Source: CAD feature listing. Evaluate the final solid. Frame: model axes, mm. Face numbers are marked on the shaded views. A direction names the side the tool comes from. Round coordinates to 2 decimals unless told otherwise and drop trailing zeros. Order: outer loops, then holes, each group sorted by start corner. A loop starts at its lowest first (then second) coordinate and runs counter-clockwise, first axis right, second up. Notation, with made-up numbers: M 41,-1 L 87,-1 A10 cw 87,13 Z; hole C 83.5,87 d6. An arc over 180 degrees is marked long. Answer in a Markdown table with one row per item. Add a question column.
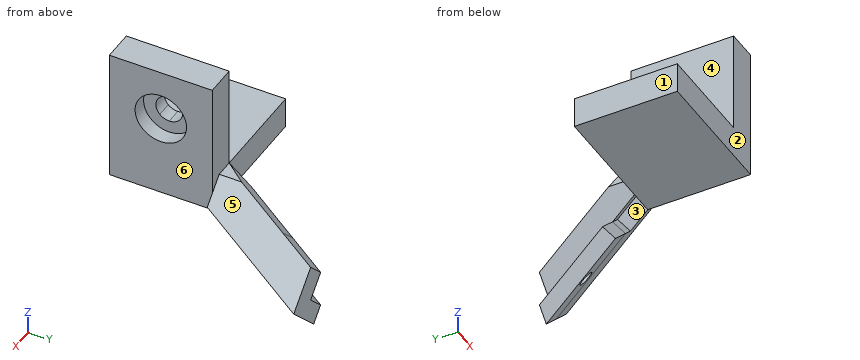
```python
from build123d import *

# Parameters (mm, degrees)
EXTRUDE_2_DEPTH     = 20
CUT_EXTRUDE_1_DEPTH = 20
SKETCH_3_R          = 5
CUT_EXTRUDE_2_DEPTH = 3
SKETCH_4_W          = 6
SKETCH_4_H          = 6
EXTRUDE_3_DEPTH     = 84
CUT_EXTRUDE_3_DEPTH = 84
CUT_EXTRUDE_4_DEPTH = 84
CUT_EXTRUDE_5_DEPTH = 84
SKETCH_9_R          = 1.5
EXTRUDE_4_DEPTH     = 3
CUT_EXTRUDE_6_DEPTH = 6
CUT_EXTRUDE_7_DEPTH = 2.5


with BuildPart() as part:
    # 草图1 → 凸台-拉伸2 (new body)
    with BuildSketch(Plane(origin=(0, 0, 0), x_dir=(1, 0, 0), z_dir=(0, 1, 0))):
        Polygon((0, 0), (0, -20), (6, -20), (6, 6), (-20, 6), (-20, 0), align=None)
    extrude(amount=EXTRUDE_2_DEPTH)

    # 草图2 → 切除-拉伸1 (cut)
    with BuildSketch(Plane(origin=(6, 0, 0), x_dir=(0, 0, -1), z_dir=(1, 0, 0))):
        with BuildLine():
            ThreePointArc((-11.838477631, 11.838477631), (-11.838477631, 8.161522369), (-8.161522369, 8.161522369))
            Line((-8.161522369, 8.161522369), (-11.838477631, 11.838477631))
        make_face()
        with BuildLine():
            Line((-11.838477631, 11.838477631), (-8.161522369, 8.161522369))
            ThreePointArc((-8.161522369, 8.161522369), (-7.597913215, 9.005023076), (-7.4, 10))
            ThreePointArc((-7.4, 10), (-9.005023076, 12.402086785), (-11.838477631, 11.838477631))
        make_face()
    extrude(amount=-CUT_EXTRUDE_1_DEPTH, mode=Mode.SUBTRACT)

    # 草图3 → 切除-拉伸2 (cut)
    with BuildSketch(Plane(origin=(6, 0, 0), x_dir=(0, 0, -1), z_dir=(1, 0, 0))):
        with Locations((-10, 10)):
            Circle(SKETCH_3_R)
    extrude(amount=-CUT_EXTRUDE_2_DEPTH, mode=Mode.SUBTRACT)

    # 草图4 → 凸台-拉伸3 (add)
    with BuildSketch(Plane(origin=(0, 20, 0), x_dir=(1, 0, 0), z_dir=(0, 1, 0))):
        Polygon((65.39696962, 65.39696962), (6, 6), (7.767766953, 4.232233047), (67.164736573, 63.629202667), align=None)
        Polygon((4.232233047, 7.767766953), (6, 6), (65.39696962, 65.39696962), (63.629202667, 67.164736573), align=None)
        Polygon((0, 6), (6, 6), (4.232233047, 7.767766953), (0, 12), align=None)
        with Locations((3, 3)):
            Rectangle(SKETCH_4_W, SKETCH_4_H)
        Polygon((7.767766953, 4.232233047), (6, 6), (6, 0), (12, 0), align=None)
    extrude(amount=EXTRUDE_3_DEPTH)

    # 草图5 → 切除-拉伸3 (cut)
    with BuildSketch(Plane(origin=(-1.767766953, 0, -1.767766953), x_dir=(-0.7071067811865438, 0, 0.7071067811865513), z_dir=(-0.7071067811865513, 0, -0.7071067811865438))):
        Polygon((-8.485281374, 104), (-92.485281374, 104), (-92.485281374, 20), (-8.485281374, 20), (-20.985281374, 41.650635095), (-12.5, 41.650635095), (-8.485281374, 34.696938457), align=None)
        Polygon((0, 104), (-8.485281374, 104), (-8.485281374, 34.696938457), (0, 20), align=None)
    extrude(amount=-CUT_EXTRUDE_3_DEPTH, mode=Mode.SUBTRACT)

    # 草图6 → 切除-拉伸4 (cut)
    with BuildSketch(Plane(origin=(1.767766953, 0, 1.767766953), x_dir=(0.7071067811865438, 0, -0.7071067811865513), z_dir=(0.7071067811865513, 0, 0.7071067811865438))):
        Polygon((8.485281374, 34.696938457), (8.485281374, 20), (0, 20), align=None)
    extrude(amount=CUT_EXTRUDE_4_DEPTH, mode=Mode.SUBTRACT)

    # 草图7 → 切除-拉伸5 (cut)
    with BuildSketch(Plane(origin=(-1.767766953, 0, -1.767766953), x_dir=(-0.7071067811865438, 0, 0.7071067811865513), z_dir=(-0.7071067811865513, 0, -0.7071067811865438))):
        Polygon((-8.485281374, 20), (-2.5, 20), (-2.5, 24.330127019), (-2.5, 104), (-8.485281374, 104), (-8.485281374, 34.696938457), align=None)
        Polygon((-2.5, 24.330127019), (-2.5, 20), (0, 20), align=None)
    extrude(amount=CUT_EXTRUDE_5_DEPTH, mode=Mode.SUBTRACT)

    # 草图9 → 凸台-拉伸4 (add)
    with BuildSketch(Plane(origin=(-1.623724357, 1.325765386, 1.623724357), x_dir=(-0.47434164902525855, 0.3872983346207449, -0.7905694150420924), z_dir=(0.6123724356957914, -0.5, -0.6123724356957978))):
        Polygon((23.059741154, 40.529312363), (27.531877109, 38.293244386), (18.587605199, 20.404700566), (14.115469244, 22.640768543), align=None)
        with Locations(Location((20.823673176, 30.467006465, 0), (0, 0, 333.434948823))):
            Circle(SKETCH_9_R, mode=Mode.SUBTRACT)
    extrude(amount=-EXTRUDE_4_DEPTH)

    # 草图10 → 切除-拉伸6 (cut)
    with BuildSketch(Plane(origin=(-1.767766953, 0, -1.767766953), x_dir=(0.7071067811865438, 0, -0.7071067811865512), z_dir=(0.7071067811865512, 0, 0.7071067811865438))):
        Polygon((17.521179759, 41.650635095), (20.985281374, 41.650635095), (18.387205163, 43.150635095), align=None)
    extrude(amount=-CUT_EXTRUDE_6_DEPTH, mode=Mode.SUBTRACT)

    # 草图11 → 切除-拉伸7 (cut)
    with BuildSketch(Plane(origin=(-1.767766953, 0, -1.767766953), x_dir=(-0.7071067811865438, 0, 0.7071067811865513), z_dir=(-0.7071067811865513, 0, -0.7071067811865438))):
        Polygon((-8.387205163, 25.830127019), (-5.021179759, 20), (-8.485281374, 20), (-10.985281374, 24.330127019), align=None)
    extrude(amount=-CUT_EXTRUDE_7_DEPTH, mode=Mode.SUBTRACT)


solid = part.part
```
(1) Cut plane A-A (z = 10). Return loops of the section in (x, y), and give its area (3 significant figures).
(2) Cut plane D-D (z = 16.5). Return loops of the section in (x, y).
(3) Cut plane B-B (y = 22.5). Return loops of the section in (x, z), and give its area (3 significant figures).
(4) Line query: line 1 (Y direction, x = 4.3, z = 10); line 2 (X direction, y = 18, z = -0.5); line 3 (Z direction, x = -8, y = 3). Output: solid intervals per line, ascending. Write a range as from..to.
(5) Pin query (flat end, axial travel): pin 1 (22 mm diameter, centred on y = 6, z = 14, fed in from -X); pin 2 (22 mm diameter, centred on y = 10, z = 6.5, fed in from +X); pin 3 (1.8 mm diameter, centred on x = 2, z = 8.5, fed in from +Y); pin 4 (8 mm diameter, centred on x = -1.5, y = 5.5, fed in from +Z). Return the tip coordinate at first contact, or that it passes through.
(6) Access query for the marked faces 4, 5 and 6. Directions: +Z, -Z, +X, -X, +Y, -Y. A direction counts if a zero-diameter tool reaches every point of the face in a straight line with its end or side. Return the directions, or none.
(7) Cut plane C-C (x = -4). Return loops of the section in (y, z).
(8) Draft query along Y for the marked faces 1, 2 and 3. Return one class per face: +Y half, -Y half, draft (parallel to the pull), parting line (faces both ways), or undercut.
Answer list:
| question | item | result |
|---|---|---|
| 1 | outline | M 0,0 L 6,0 L 6,5 L 3,5 L 3,7.4 L 0,7.4 Z; M 0,12.6 L 3,12.6 L 3,15 L 6,15 L 6,20 L 0,20 Z |
| 1 | area | 74.4 mm² |
| 2 | outline | M 0,0 L 6,0 L 6,20 L 0,20 Z |
| 3 | outline | M 0,-3.54 L 2.8,-6.34 L 4.57,-4.57 L 7.02,-7.02 L 8.79,-5.25 L 3.54,0 L 2.04,0 L 0,-2.04 Z |
| 3 | area | 32.6 mm² |
| 4 | line 1 | 0..5, 15..20 |
| 4 | line 2 | -20..6 |
| 4 | line 3 | -6..0 |
| 5 | pin 1 | x = 0 |
| 5 | pin 2 | x = 6 |
| 5 | pin 3 | y = 20 |
| 5 | pin 4 | z = 20 |
| 6 | face 4 | +Z, -X, +Y, -Y |
| 6 | face 5 | +Z, +X, +Y |
| 6 | face 6 | +Z, -Z, +X, -Y |
| 7 | outline | M 0,-6 L 20,-6 L 20,0 L 0,0 Z |
| 8 | face 1 | draft |
| 8 | face 2 | -Y half |
| 8 | face 3 | undercut |
